For this review, take the finished solid that the model builds, in its own axes (mm). A direction names the side the tool comes from. Give positions to 0.01 mm unless a question says otherwise; leave off trailing zeros. Write each loop counter-clockwise with the first axis right and the second up, starting at its lowest first coordinate (ties: lowest second). Pieces come first, ordered by that corner, then holes. Notation, with made-up numbers: (68, -10) -> (83, -10) arc R11 cw to (83, 2) -> close; hole circle Ø1 at (70, -4). An arc over 180 degrees is marked (long way). Return JSON: item names as keys, results as strings.
from build123d import *

# Parameters (mm, degrees)
SKETCH3_R           = 88.9
BOSS_EXTRUDE2_DEPTH = 15.24
SKETCH1_R           = 76.2
SKETCH1_R_2         = 50.8
CUT_EXTRUDE1_DEPTH  = 12.7
SKETCH4_R           = 3.175
SKETCH4_R_2         = 50.8
CUT_EXTRUDE3_DEPTH  = 127.643900761


with BuildPart() as part:
    # Sketch3 → Boss-Extrude2 (new body)
    with BuildSketch(Plane.XY):
        with Locations(Location((0, 0, 0), (0, 0, 180))):
            Circle(SKETCH3_R)
    extrude(amount=BOSS_EXTRUDE2_DEPTH)

    # Sketch1 → Cut-Extrude1 (cut)
    with BuildSketch(Plane.XY):
        Circle(SKETCH1_R)
        Circle(SKETCH1_R_2, mode=Mode.SUBTRACT)
    extrude(amount=CUT_EXTRUDE1_DEPTH, mode=Mode.SUBTRACT)

    # Sketch4 → Cut-Extrude3 (cut, through all)
    with BuildSketch(Plane.XY):
        with Locations(Location((-63.5, 0, 0), (0, 0, 180))):
            Circle(SKETCH4_R)
        with Locations(Location((0, 0, 0), (0, 0, 180))):
            Circle(SKETCH4_R_2)
        with Locations(Location((-60.678873167, 18.716953575, 0), (0, 0, 180))):
            Circle(SKETCH4_R)
        with Locations(Location((-52.466162169, 35.770823687, 0), (0, 0, 180))):
            Circle(SKETCH4_R)
        with Locations(Location((-39.591602418, 49.646299137, 0), (0, 0, 180))):
            Circle(SKETCH4_R)
        with Locations(Location((-23.199155047, 59.110483039, 0), (0, 0, 180))):
            Circle(SKETCH4_R)
        with Locations(Location((-4.745360943, 63.322441121, 0), (0, 0, 180))):
            Circle(SKETCH4_R)
        with Locations(Location((14.130079306, 61.907922424, 0), (0, 0, 180))):
            Circle(SKETCH4_R)
        with Locations(Location((31.75, 54.99261314, 0), (0, 0, 180))):
            Circle(SKETCH4_R)
        with Locations(Location((46.548793861, 43.190968848, 0), (0, 0, 180))):
            Circle(SKETCH4_R)
        with Locations(Location((57.211523112, 27.551617434, 0), (0, 0, 180))):
            Circle(SKETCH4_R)
        with Locations(Location((62.790757465, 9.464183902, 0), (0, 0, 180))):
            Circle(SKETCH4_R)
        with Locations(Location((62.790757465, -9.464183902, 0), (0, 0, 180))):
            Circle(SKETCH4_R)
        with Locations(Location((57.211523112, -27.551617434, 0), (0, 0, 180))):
            Circle(SKETCH4_R)
        with Locations(Location((46.548793861, -43.190968848, 0), (0, 0, 180))):
            Circle(SKETCH4_R)
        with Locations(Location((31.75, -54.99261314, 0), (0, 0, 180))):
            Circle(SKETCH4_R)
        with Locations(Location((14.130079306, -61.907922424, 0), (0, 0, 180))):
            Circle(SKETCH4_R)
        with Locations(Location((-4.745360943, -63.322441121, 0), (0, 0, 180))):
            Circle(SKETCH4_R)
        with Locations(Location((-23.199155047, -59.110483039, 0), (0, 0, 180))):
            Circle(SKETCH4_R)
        with Locations(Location((-39.591602418, -49.646299137, 0), (0, 0, 180))):
            Circle(SKETCH4_R)
        with Locations(Location((-52.466162169, -35.770823687, 0), (0, 0, 180))):
            Circle(SKETCH4_R)
        with Locations(Location((-60.678873167, -18.716953575, 0), (0, 0, 180))):
            Circle(SKETCH4_R)
    extrude(amount=CUT_EXTRUDE3_DEPTH, mode=Mode.SUBTRACT)


solid = part.part
1. For pin 1 (2 mm diameter, centred on x = 27.5, z = 8, fed in from -Y); pin 2 (8.5 mm diameter, centred on x = -63.5, y = 0, fed in from -Z); pin 3 (2 mm diameter, centred on y = 4.5, z = 7.5, fed in from -X), all flat-tipped, find the tip position at first contact; note any pin that passes through.
Results found:
{"pin 1": "stops at y = -84.86", "pin 2": "stops at z = 12.7", "pin 3": "stops at x = -88.83"}
2. For faces 1 (the cylindrical face through (-22.51, 62.21, 13.95)), 2 (the cylindrical face through (-60.47, -46.367, 6.261)), list the 3-axis set-ups (+Z, -Z, +X, -X, +Y, -Y) from which the entire face can be reached by the end or side of a thin tool; tool diameter is ignored.
Results found:
{"face 1": "+Z, -Z", "face 2": "-Z"}
3. Add section B-B, the plane x = 0.5. State the section outline as (y, z) points.
Results found:
{"outline": "(-88.9, 0) -> (-76.2, 0) -> (-76.2, 12.7) -> (-50.8, 12.7) -> (-50.8, 15.24) -> (-88.9, 15.24) -> close; (50.8, 12.7) -> (76.2, 12.7) -> (76.2, 0) -> (88.9, 0) -> (88.9, 15.24) -> (50.8, 15.24) -> close"}
4. The part is to be moulded in two halves that separate along X. For faces 3 (the cylindrical face through (-59.991, 21.816, 13.952)), 4 (the flat face through (-65.4, -39.9, 0)), say which applies: +X half, -X half, draft (parallel to the pull), parting line (faces both ways), or undercut.
Results found:
{"face 3": "undercut", "face 4": "draft"}
5. Add section D-D, the plane x = 31.75. State the section outline as (y, z) points.
Results found:
{"outline": "(-83.04, 0) -> (-69.27, 0) -> (-69.27, 12.7) -> (-58.17, 12.7) -> (-58.17, 15.24) -> (-83.04, 15.24) -> close; (-51.82, 12.7) -> (-39.66, 12.7) -> (-39.66, 15.24) -> (-51.82, 15.24) -> close; (39.66, 12.7) -> (51.82, 12.7) -> (51.82, 15.24) -> (39.66, 15.24) -> close; (58.17, 12.7) -> (69.27, 12.7) -> (69.27, 0) -> (83.04, 0) -> (83.04, 15.24) -> (58.17, 15.24) -> close"}
6. Add section C-C, the plane z = 4.25. State the section outline as (x, y) points, plus the area to 3 significant figures.
Results found:
{"outline": "circle Ø177.8 at (0, 0); hole circle Ø152.4 at (0, 0)", "area": "6,590 mm²"}
7. Add section A-A, the plane y = 0. State the section outline as (x, z) points (3 decimals), plus the area to 3 significant figures.
Results found:
{"outline": "(-88.9, 0) -> (-76.2, 0) -> (-76.2, 12.7) -> (-66.675, 12.7) -> (-66.675, 15.24) -> (-88.9, 15.24) -> close; (-60.325, 12.7) -> (-50.8, 12.7) -> (-50.8, 15.24) -> (-60.325, 15.24) -> close; (50.8, 12.7) -> (76.2, 12.7) -> (76.2, 0) -> (88.9, 0) -> (88.9, 15.24) -> (50.8, 15.24) -> close", "area": "500 mm²"}
8. To check wall thickness, follow probe 1 along X at (y, z) = (41.5, 13); probe 2 along Y at (x, z) = (-63.5, 14.3) (3 decimals); probe 3 along Z at (x, y) = (43, 43). State the ranges of each line that lie inside material, in increasing order.
Results found:
{"probe 1": "x = -78.62 to -29.3, 29.3 to 43.86, 49.24 to 78.62", "probe 2": "y = -62.217 to -20.174, -17.26 to -3.175, 3.175 to 17.26, 20.174 to 62.217", "probe 3": "z = 12.7 to 15.24"}
